Part model, mm, in its own coordinate system. Give positions to 0.01 mm unless a question says otherwise; leave off trailing zeros. Order: outer loops, then holes, each group sorted by start corner. A loop starts at its lowest first (then second) coordinate and runs counter-clockwise, first axis right, second up.
1. Probe line 1 (Z direction, x = 113.5, y = 0.35); line 2 (Z direction, x = 116.5, y = 0.2); line 3 (X direction, y = 1.8, z = -22). List the from-to ranges inside material, lowest first.
2. Slice it at C-C on x = -44. List the corners of the cut face in (y, z), and give its area (3 significant figures).
3. Slice it at D-D on z = 51. List the corners of the cut face in (x, y), and give its area (3 significant figures).
4. Slice it at B-B on z = -9.5. List the corners of the cut face in (x, y), and give its area (3 significant figures).
5. Slice it at A-A on x = 32. List the corners of the cut face in (y, z).
6. Drop a flat-ended pin along its axis: pin 1 Ø24 at (x, z) = (32, -18.88) entering from +Y. Give the stop position or say it passes through.
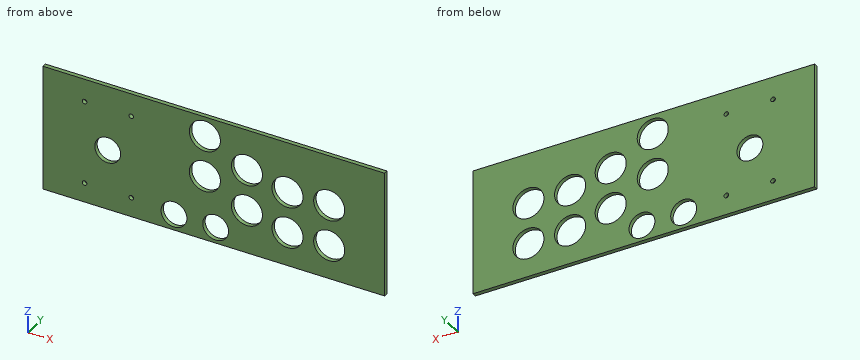
Autodesk Inventor part; units mm, degrees
ref_plane "YZ Plane" through (0, 0, 0) normal (1, 0, 0) x (0, 1, 0)
ref_plane "XZ Plane" through (0, 0, 0) normal (0, 1, 0) x (-1, 0, 0)
ref_plane "XY Plane" through (0, 0, 0) normal (0, 0, 1) x (1, 0, 0)
sketch "Sketch1" plane through (0, 0, 0) normal (0, 1, 0) x (-1, 0, 0)
  line L0 (165, 61) -> (-165, 61)
  line L1 (-165, 61) -> (-165, -61)
  line L2 (-165, -61) -> (165, -61)
  line L3 (165, -61) -> (165, 61)
  point P0 (0, 0)
  point P1 (0, -61)
  point P2 (165, 0)
  dimension "d0" = 122
  dimension "d1" = 330
extrude "Extrusion1" add sketch "Sketch1" along normal blind 4
sketch "Esboço2" plane through (0, 0, 0) normal (0, -1, 0) x (1, 0, 0)
  circle A0 centre (111.4577, -28.224) radius 15
  circle A1 centre (71.1891, -28.224) radius 15
  circle A2 centre (71.1891, 11.776) radius 15
  circle A3 centre (111.4577, 11.776) radius 15
  circle A4 centre (31.9991, -18.8759) radius 15
  circle A5 centre (31.9991, 21.1241) radius 15
  circle A6 centre (-8.629, 1.9775) radius 15
  circle A7 centre (-8.629, 41.9775) radius 15
  circle A8 centre (1.7977, -45.4819) radius 12.5
  circle A9 centre (-38.4709, -45.4819) radius 12.5
  circle A10 centre (-102.5005, -2.2868) radius 12.5
  circle A11 centre (-79.7133, -42.1687) radius 2.25
  circle A12 centre (-124.8372, -42.1687) radius 2.25
  circle A13 centre (-79.7133, 38.8141) radius 2.1608
  circle A14 centre (-124.8372, 38.8141) radius 2.25
  point P0 (0, 0)
  dimension "d4" = 30
  dimension "d5" = 30
  dimension "d6" = 30
  dimension "d7" = 30
  dimension "d8" = 30
  dimension "d9" = 30
  dimension "d10" = 40
  dimension "d11" = 40
  dimension "d12" = 40
  dimension "d13" = 30
  dimension "d14" = 30
  dimension "d15" = 40
  dimension "d16" = 25
  dimension "d17" = 25
  dimension "d18" = 25
  dimension "d19" = 4.5
  dimension "d20" = 4.5
  dimension "d21" = 4.5
extrude "Extrusão2" cut sketch "Esboço2" against normal blind 5
sketch "Esboço3" plane through (0, 0, 0) normal (0, -1, 0) x (1, 0, 0)
  point P0 (0, 0)
properties part number "controles2"
Data:
1. line 1: z = -61 to -43.08, -13.36 to -3.08, 26.64 to 61
1. line 2: z = -61 to -42.35, -14.1 to -2.35, 25.9 to 61
1. line 3: x = -165 to 17.33, 46.67 to 57.54, 84.84 to 97.81, 125.11 to 165
2. outline: (0, -61) - (4, -61) - (4, -56.69) - (0, -56.69) - close; (0, -34.27) - (4, -34.27) - (4, 61) - (0, 61) - close
2. area: 398 mm2
3. outline: (-165, 0) - (-20.61, 0) - (-20.61, 4) - (-165, 4) - close; (3.35, 0) - (165, 0) - (165, 4) - (3.35, 4) - close
3. area: 1,220 mm2
4. outline: (-165, 0) - (-112.71, 0) - (-112.71, 4) - (-165, 4) - close; (-92.29, 0) - (-18.29, 0) - (-18.29, 4) - (-92.29, 4) - close; (1.03, 0) - (20.29, 0) - (20.29, 4) - (1.03, 4) - close; (43.71, 0) - (165, 0) - (165, 4) - (43.71, 4) - close
4. area: 1,070 mm2
5. outline: (0, -61) - (4, -61) - (4, -33.88) - (0, -33.88) - close; (0, -3.88) - (4, -3.88) - (4, 6.12) - (0, 6.12) - close; (0, 36.12) - (4, 36.12) - (4, 61) - (0, 61) - close
6. pin 1: passes through
